For this review, take the finished solid that the model builds, in its own axes (mm). Face numbers are marked on the shaded views. A direction names the side the tool comes from. Give positions to 0.01 mm unless a question says otherwise; leave off trailing zeros. Order: outer loops, then holes, each group sorted by start corner. A loop starts at its lowest first (then second) coordinate and runs counter-clockwise, first axis right, second up. Notation, with made-up numbers: (-13.5, -24) - (22.5, -24) arc R21 cw to (22.5, -5) - close; hole circle Ø2 at (-1, 53.5). An arc over 180 degrees is marked (long way). Use a Markdown table: item, result. Add a question column.
1) Clearance check with flat-ended pins moving along their axes: P1, Ø1, axis at x = -88, y = 104.5, coming from the -Z side; P2, Ø12, axis at y = 58.5, z = 164, coming from the -X side; P3, Ø7.5, axis at x = 68.5, z = 113, coming from the +Y side. State where each tip first meets the part, or that it passes through.
2) Mouldability with a two-part tool opening along Y and no side actions: class the marked faces 4, 5, 6 and 7 as released by +Y, released by -Y, zero draft, split by the parting line, or undercut.
3) Wall thickness on L1, parallel to Y at x = 0, z = 63.5; L2, parallel to Z at x = 154.5, y = 76; L3, parallel to X at y = 16, z = -93: over which ranges is each line inside the solid? List them lowest first.
4) We need section A-A on z = 175.5. Write out the cut boundary in (x, y).
5) We need section C-C on x = 0. Write out the cut boundary in (y, z), then the cut area to 3 significant figures.
6) We need section D-D on y = -178. Write out the cut boundary in (x, z), then the cut area to 3 significant figures.
7) We need section B-B on z = 111. Write out the cut boundary in (x, y), then the cut area to 3 significant figures.
8) Machinability: for the marked faces 1, 2 and 3, which of the approach directions +Z, -Z, +X, -X, +Y, -Y give a long, thin tool a straight path to every point of the face, cutting with its end or side? Answer none if there is none.
```python
from build123d import *

# Parameters (mm, degrees)
F0_W      = 235.571132
F0_H      = 204.806238
F0_R      = 46.940365
F1_DEPTH  = 25.4
F2_R      = 62.434365
F2_R_2    = 46.940365
F3_DEPTH  = 76.2
F4_W      = 371.668696
F4_H      = 250.246078
F4_R      = 10.18532
F4_R_2    = 71.315822
F5_DEPTH  = 25.4
F6_R      = 48.285319
F6_R_2    = 10.18532
F6_R_3    = 124.655822
F6_R_4    = 71.315822
F7_DEPTH  = 101.6
F8_W      = 767.606258
F8_H      = 524.892748
F8_R      = 35.842084
F8_R_2    = 31.200306
F9_DEPTH  = 25.4
F10_R     = 79.460308
F10_R_2   = 31.200306
F10_R_3   = 122.202093
F10_R_4   = 35.842084
F11_DEPTH = 127


with BuildPart() as f1:
    # F0 (on Top) → F1 (new body)
    with BuildSketch(Plane.XY):
        Rectangle(F0_W, F0_H)
        Circle(F0_R, mode=Mode.SUBTRACT)
    extrude(amount=F1_DEPTH)

    # F2 (on face) → F3 (join)
    with BuildSketch(Plane.XY.offset(25.4)):
        Circle(F2_R)
        Circle(F2_R_2, mode=Mode.SUBTRACT)
    extrude(amount=F3_DEPTH)

    # F4 (on face) → F5 (join)
    with BuildSketch(Plane.XY.offset(101.6)):
        Rectangle(F4_W, F4_H)
        with Locations((-97.129136, 0)):
            Circle(F4_R, mode=Mode.SUBTRACT)
        with Locations((91.415659, 0)):
            Circle(F4_R_2, mode=Mode.SUBTRACT)
    extrude(amount=F5_DEPTH)

    # F6 (on face) → F7 (join)
    with BuildSketch(Plane.XY.offset(127)):
        with Locations((-97.129136, 0)):
            Circle(F6_R)
        with Locations((-97.129136, 0)):
            Circle(F6_R_2, mode=Mode.SUBTRACT)
        with Locations((91.415659, 0)):
            Circle(F6_R_3)
        with Locations((91.415659, 0)):
            Circle(F6_R_4, mode=Mode.SUBTRACT)
    extrude(amount=F7_DEPTH)

    # F8 (on face) → F9 (join)
    with BuildSketch(Plane(origin=(0, 0, 0), x_dir=(1, 0, 0), z_dir=(0, 0, -1))):
        Rectangle(F8_W, F8_H)
        with Locations((-249.21973, 3.120291)):
            Circle(F8_R, mode=Mode.SUBTRACT)
        with Locations((265.806586, 1.147008)):
            Circle(F8_R_2, mode=Mode.SUBTRACT)
    extrude(amount=F9_DEPTH)

    # F10 (on face) → F11 (join)
    with BuildSketch(Plane(origin=(0, 0, -25.4), x_dir=(1, 0, 0), z_dir=(0, 0, -1))):
        with Locations((265.806586, 1.147008)):
            Circle(F10_R)
        with Locations((265.806586, 1.147008)):
            Circle(F10_R_2, mode=Mode.SUBTRACT)
        with Locations((-249.21973, 3.120291)):
            Circle(F10_R_3)
        with Locations((-249.21973, 3.120291)):
            Circle(F10_R_4, mode=Mode.SUBTRACT)
    extrude(amount=F11_DEPTH)


solid = f1.part
```
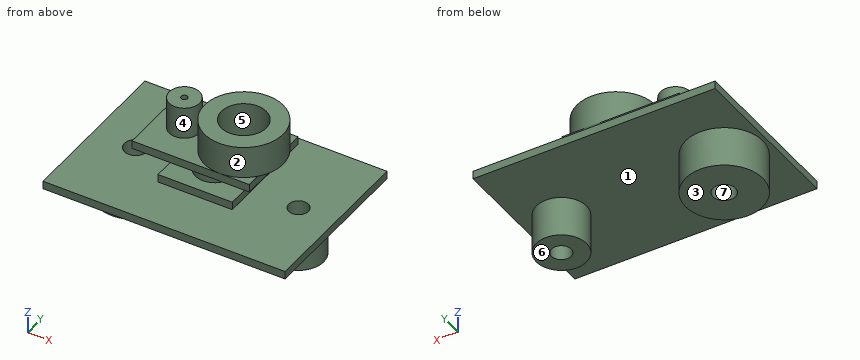
Checked values:
| question | item | result |
|---|---|---|
| 1 | P1 | z = -25.4 |
| 1 | P2 | x = -21.65 |
| 1 | P3 | y = 125.12 |
| 2 | face 4 | split by the parting line |
| 2 | face 5 | undercut |
| 2 | face 6 | zero draft |
| 2 | face 7 | undercut |
| 3 | L1 | -62.43 to -46.94, 46.94 to 62.43 |
| 3 | L2 | -25.4 to 0, 101.6 to 228.6 |
| 3 | L3 | -369.92 to -279.54, -218.9 to -128.52, 188.22 to 239.74, 291.87 to 343.39 |
| 4 | outline | circle Ø96.57 at (-97.13, 0); circle Ø249.31 at (91.42, 0); hole circle Ø20.37 at (-97.13, 0); hole circle Ø142.63 at (91.42, 0) |
| 5 | outline | (-262.45, -25.4) - (262.45, -25.4) - (262.45, 0) - (102.4, 0) - (102.4, 25.4) - (62.43, 25.4) - (62.43, 101.6) - (125.12, 101.6) - (125.12, 127) - (84.75, 127) - (84.75, 228.6) - (-84.75, 228.6) - (-84.75, 127) - (-125.12, 127) - (-125.12, 101.6) - (-62.43, 101.6) - (-62.43, 25.4) - (-102.4, 25.4) - (-102.4, 0) - (-262.45, 0) - close; hole (-46.94, 0) - (46.94, 0) - (46.94, 101.6) - (-46.94, 101.6) - close |
| 5 | area | 42,100 mm² |
| 6 | outline | (-383.8, -25.4) - (383.8, -25.4) - (383.8, 0) - (-383.8, 0) - close |
| 6 | area | 19,500 mm² |
| 7 | outline | (-185.83, -125.12) - (185.83, -125.12) - (185.83, 125.12) - (-185.83, 125.12) - close; hole circle Ø20.37 at (-97.13, 0); hole circle Ø142.63 at (91.42, 0) |
| 7 | area | 76,700 mm² |
| 8 | face 1 | -Z |
| 8 | face 2 | +Z |
| 8 | face 3 | -Z, +X, -X, +Y, -Y |
